from build123d import *

# Parameters (mm, degrees)
F1_DEPTH = 45
F2_SIZE  = 10
F4_D     = 5.8
F6_DEPTH = 60.001


with BuildPart() as f1:
    # F0 (on Right) → F1 (new body, symmetric)
    with BuildSketch(Plane.YZ):
        with BuildLine():
            Line((83, 0), (0, 0))
            Line((0, 0), (0, -6.35))
            Line((0, -6.35), (82.65, -6.35))
            ThreePointArc((82.65, -6.35), (86.8926406871, -8.1073593129), (88.65, -12.35))
            Line((88.65, -12.35), (88.65, -48))
            ThreePointArc((88.65, -48), (92.1647186258, -56.4852813742), (100.65, -60))
            Line((100.65, -60), (150, -60))
            Line((150, -60), (150, -53.65))
            Line((150, -53.65), (101, -53.65))
            ThreePointArc((101, -53.65), (96.7573593129, -51.8926406871), (95, -47.65))
            Line((95, -47.65), (95, -12))
            ThreePointArc((95, -12), (91.4852813742, -3.5147186258), (83, 0))
        make_face()
    extrude(amount=F1_DEPTH, both=True)

    # F2
    f2_edges = [f1.edges().sort_by_distance(p)[0] for p in [
        (45, 0, -3.175),
        (-45, 0, -3.175),
    ]]
    chamfer(f2_edges, length=F2_SIZE)

    # F4 (through all)
    with Locations(Plane.XY):
        with Locations((-15, 5), (-15, 65), (15, 65), (15, 5)):
            Hole(F4_D / 2)

    # F5 (on face) → F6 (cut, through all)
    with BuildSketch(Plane(origin=(0, 0, -60), x_dir=(1, 0, 0), z_dir=(0, 0, -1))):
        with BuildLine():
            ThreePointArc((31, -113), (25, -107), (19, -113))
            Line((19, -113), (19, -125))
            Line((19, -125), (19, -137))
            ThreePointArc((19, -137), (25, -143), (31, -137))
            Line((31, -137), (31, -125))
            Line((31, -125), (31, -113))
        make_face()
        with BuildLine():
            Line((-31, -125), (-31, -137))
            ThreePointArc((-31, -137), (-25, -143), (-19, -137))
            Line((-19, -137), (-19, -125))
            Line((-19, -125), (-19, -113))
            ThreePointArc((-19, -113), (-25, -107), (-31, -113))
            Line((-31, -113), (-31, -125))
        make_face()
    extrude(amount=-F6_DEPTH, mode=Mode.SUBTRACT)


solid = f1.part
Geometry: final body of the model. Coordinates: model frame, mm. A direction names the side the tool comes from. Coordinates: 2 decimals unless noted, no trailing zeros. Write each loop counter-clockwise with the first axis right and the second up, starting at its lowest first coordinate (ties: lowest second). Pieces come first, ordered by that corner, then holes. Notation, with made-up numbers: (-33, 87) - (-3, 87) arc R15 cw to (-3, 108) - close; hole circle Ø7 at (88.5, 84). An arc over 180 degrees is marked (long way). Return JSON: item names as keys, results as strings.
Item 1: Pin query (flat end, axial travel): pin 1 Ø12 at (x, z) = (13, -33.5) entering from +Y; pin 2 Ø3 at (x, z) = (26, -40.5) entering from -Y; pin 3 Ø7.5 at (x, y) = (15, 5) entering from -Z. Return the tip coordinate at first contact, or that it passes through.
Completed:
{"pin 1": "stops at y = 95", "pin 2": "stops at y = 88.65", "pin 3": "stops at z = -6.35"}
Item 2: Section query C-C (x = 15). Output: boundary loops of the cut face in (y, z), and give its area (3 significant figures).
Completed:
{"outline": "(0, -6.35) - (2.1, -6.35) - (2.1, 0) - (0, 0) - close; (7.9, -6.35) - (62.1, -6.35) - (62.1, 0) - (7.9, 0) - close; (67.9, -6.35) - (82.65, -6.35) arc R6 cw to (88.65, -12.35) - (88.65, -48) arc R12 ccw to (100.65, -60) - (150, -60) - (150, -53.65) - (101, -53.65) arc R6 cw to (95, -47.65) - (95, -12) arc R12 ccw to (83, 0) - (67.9, 0) - close", "area": "1,170 mm2"}
Item 3: Section query D-D (z = -55.5). Output: boundary loops of the cut face in (x, y), and give its area (3 significant figures).
Completed:
{"outline": "(-45, 91.28) - (45, 91.28) - (45, 150) - (-45, 150) - close; hole (-31, 113) arc R6 ccw to (-19, 113) - (-19, 137) arc R6 ccw to (-31, 137) - close; hole (19, 113) arc R6 ccw to (31, 113) - (31, 137) arc R6 ccw to (19, 137) - close", "area": "4,480 mm2"}
Item 4: Line query: L1, parallel to Y at x = -15, z = -4; L2, parallel to Y at x = -15, z = -1.75; L3, parallel to Z at x = -41, y = 100.5. Output: solid intervals per line, ascending.
Completed:
{"L1": "y = 0 to 2.1, 7.9 to 62.1, 67.9 to 91.94", "L2": "y = 0 to 2.1, 7.9 to 62.1, 67.9 to 89.24", "L3": "z = -60 to -53.63"}
Item 5: Section query B-B (x = -25). Output: boundary loops of the cut face in (y, z).
Completed:
{"outline": "(0, -6.35) - (82.65, -6.35) arc R6 cw to (88.65, -12.35) - (88.65, -48) arc R12 ccw to (100.65, -60) - (107, -60) - (107, -53.65) - (101, -53.65) arc R6 cw to (95, -47.65) - (95, -12) arc R12 ccw to (83, 0) - (0, 0) - close; (143, -60) - (150, -60) - (150, -53.65) - (143, -53.65) - close"}
Item 6: Section query A-A (y = 5). Output: boundary loops of the cut face in (x, z), and give its area (3 significant figures).
Completed:
{"outline": "(-40, -6.35) - (-17.9, -6.35) - (-17.9, 0) - (-40, 0) - close; (-12.1, -6.35) - (12.1, -6.35) - (12.1, 0) - (-12.1, 0) - close; (17.9, -6.35) - (40, -6.35) - (40, 0) - (17.9, 0) - close", "area": "434 mm2"}
Item 7: Reachability of faces 5 (the face through (1, 125, -60)), 6 (the face through (45, 90, -25)), 7 (the face through (-31, 125, -57)), 8 (the face through (1, 41, -6.35)), 9 (the face through (1, 95, -30)) from +Z, -Z, +X, -X, +Y, -Y: full face, straight path, thin tool, end or side. Return the list, or none.
Completed:
{"face 5": "-Z, +X, -X, +Y, -Y", "face 6": "+Z, -Z, +X, +Y, -Y", "face 7": "+Z, -Z", "face 8": "-Z, +X, -X, -Y", "face 9": "+Z, +X, -X, +Y"}
Item 8: Pull-direction query (X, two-part tool) for faces 1 (the face through (-19, 125, -57)), 2 (the face through (40, 5, -3)), 3 (the face through (1, 126, -53.65)), 4 (the face through (-45, 90, -25)); classes: +X half, -X half, draft (parallel to the pull), parting line (faces both ways), or undercut.
Completed:
{"face 1": "undercut", "face 2": "+X half", "face 3": "draft", "face 4": "-X half"}
